from build123d import *

# Parameters (mm, degrees)
FLAT_SKETCH_R           = 19.05
FLAT_SKETCH_R_2         = 15.875
FLAT_SKETCH_R_3         = 7.62
FLAT_SKETCH_R_4         = 3.3655
EXTRUDE_FACE_DEPTH      = 3.175
FLAT_SKETCH_4_R         = 3.3655
EXTRUDE_CUT_HOLES_DEPTH = 3.175


with BuildPart() as part:
    # Flat sketch → Extrude face (new body)
    # profile 1 of 7: a face of its own
    with BuildSketch(Plane.XY):
        Circle(FLAT_SKETCH_R)
        Circle(FLAT_SKETCH_R_2, mode=Mode.SUBTRACT)
    # profile 2 of 7: a face of its own
    with BuildSketch(Plane.XY):
        with Locations((72.263, 0)):
            Circle(FLAT_SKETCH_R_3)
        with Locations((72.263, 0)):
            Circle(FLAT_SKETCH_R_4, mode=Mode.SUBTRACT)
    # profile 3 of 7: a face of its own
    with BuildSketch(Plane.XY):
        with Locations((72.263, 0)):
            Circle(FLAT_SKETCH_R_4)
    # profile 4 of 7: a face of its own
    with BuildSketch(Plane.XY):
        with BuildLine():
            Line((73.468272408, 7.524075918), (3.013181019, 18.810189796))
            ThreePointArc((3.013181019, 18.810189796), (14.49661337, 12.359235445), (19.05, 0))
            ThreePointArc((19.05, 0), (14.49661337, -12.359235445), (3.013181019, -18.810189796))
            Line((3.013181019, -18.810189796), (73.468272408, -7.524075918))
            ThreePointArc((73.468272408, -7.524075918), (64.643, 0), (73.468272408, 7.524075918))
        make_face()
        with Locations((36.83, 0)):
            Circle(FLAT_SKETCH_R_4, mode=Mode.SUBTRACT)
        with Locations((48.641, 0)):
            Circle(FLAT_SKETCH_R_4, mode=Mode.SUBTRACT)
        with Locations((60.452, 0)):
            Circle(FLAT_SKETCH_R_4, mode=Mode.SUBTRACT)
    # profile 5 of 7: a face of its own
    with BuildSketch(Plane.XY):
        with Locations((60.452, 0)):
            Circle(FLAT_SKETCH_R_4)
    # profile 6 of 7: a face of its own
    with BuildSketch(Plane.XY):
        with Locations((48.641, 0)):
            Circle(FLAT_SKETCH_R_4)
    # profile 7 of 7: a face of its own
    with BuildSketch(Plane.XY):
        with Locations((36.83, 0)):
            Circle(FLAT_SKETCH_R_4)
    extrude(amount=EXTRUDE_FACE_DEPTH)

    # Flat sketch<4> → Extrude cut - holes (cut)
    with BuildSketch(Plane.XY):
        with Locations((72.263, 0)):
            Circle(FLAT_SKETCH_4_R)
        with Locations((60.452, 0)):
            Circle(FLAT_SKETCH_4_R)
        with Locations((48.641, 0)):
            Circle(FLAT_SKETCH_4_R)
        with Locations((36.83, 0)):
            Circle(FLAT_SKETCH_4_R)
    extrude(amount=EXTRUDE_CUT_HOLES_DEPTH, mode=Mode.SUBTRACT)


solid = part.part
Input: part model. Units: mm. Frame: model coordinates. Give positions to 0.01 mm unless a question says otherwise; leave off trailing zeros. Write each loop counter-clockwise with the first axis right and the second up, starting at its lowest first coordinate (ties: lowest second). Pieces come first, ordered by that corner, then holes. Notation, with made-up numbers: M 13.5,43.25 L 25.5,43.25 A21 ccw 25.5,82.25 Z; hole C 66,-36 d11. An arc over 180 degrees is marked long. Use one line per item in the form item = value.
1. First-contact query: P1, Ø1.5, axis at x = 26, z = 1.5, coming from the +Y side; P2, Ø7.5, axis at x = 72.263, y = 0, coming from the -Z side; P3, Ø4, axis at x = 48.641, y = 0, coming from the -Z side. Flat tips, straight axial feed; report the tip coordinate or a pass-through.
Outcome:
P1 = 15.25
P2 = 0
P3 = through
2. Mould query, pull axis Y, two halves, no side actions, for faces 1 (the face through (-19.044, 0.461, 1.565)), 2 (the face through (39.94, -1.29, 1.57)), 3 (the face through (30, 0, 0)), 4 (the face through (68.9, 0.1, 1.6)). Classes: released by +Y, released by -Y, zero draft, split by the parting line, or undercut.
Outcome:
face_1 = split by the parting line
face_2 = undercut
face_3 = zero draft
face_4 = undercut
3. Cut plane D-D on y = 13.5. Return loops of the section in (x, z) (3 decimals).
Outcome:
outline = M -13.441,0 L -8.353,0 L -8.353,3.175 L -13.441,3.175 Z; M 8.353,0 L 36.163,0 L 36.163,3.175 L 8.353,3.175 Z
4. Cut plane B-B on x = 0. Return loops of the section in (y, z) (3 decimals), and give its area (3 significant figures).
Outcome:
outline = M -19.05,0 L -15.875,0 L -15.875,3.175 L -19.05,3.175 Z; M 15.875,0 L 19.05,0 L 19.05,3.175 L 15.875,3.175 Z
area = 20.2 mm²
5. Cut plane A-A on y = 0. State how many separate pieces and enclosed holes the cut face has, and give its area (3 significant figures).
Outcome:
separate_pieces = 6
enclosed_holes = 0
area = 128 mm²
6. Ray query, L1, parallel to X at y = 2.5, z = 2.15; L2, parallel to X at y = 3, z = 0.35; L3, parallel to Y at x = 8, z = 0.6. Return the intervals inside material, ascending.
Outcome:
L1 = -18.89 to -15.68, 15.68 to 34.58, 39.08 to 46.39, 50.89 to 58.2, 62.71 to 70.01, 74.52 to 79.46
L2 = -18.81 to -15.59, 15.59 to 35.3, 38.36 to 47.12, 50.17 to 58.93, 61.98 to 70.74, 73.79 to 79.27
L3 = -18.01 to -13.71, 13.71 to 18.01
